Source: CAD feature listing. Evaluate the final solid. Frame: model axes, mm. Face numbers are marked on the shaded views. Coordinates: 2 decimals unless noted, no trailing zeros. Write item = value, one per line. Start each with the question number.
Autodesk Inventor part; units mm, degrees
ref_plane "YZ Plane" through (0, 0, 0) normal (1, 0, 0) x (0, 1, 0)
ref_plane "XZ Plane" through (0, 0, 0) normal (0, 1, 0) x (-1, 0, 0)
ref_plane "XY Plane" through (0, 0, 0) normal (0, 0, 1) x (1, 0, 0)
sketch "Esboço2" plane through (0, 0, 0) normal (0, 0, 1) x (1, 0, 0)
  line L0 (0, 0) -> (4, 0)
  line L1 (4, 0) -> (4, 4.3)
  line L2 (0, 4.3) -> (0, 0)
  arc A0 (0, 4.3) -> (4, 4.3) centre (2, 9.4235) ccw
  dimension "d0" = 4
  dimension "d1" = 4.3
  dimension "d70" = 5.5
revolve "Revolução1" add sketch "Esboço2" angle 360 about axis through (0, 0, 0) along (1, 0, 0)
sketch "Esboço11" plane through (4, 0, 0) normal (1, 0, 0) x (0, 0, -1)
  circle A0 centre (0, 0) radius 2.55
  circle A1 centre (0, 0) radius 2.95
  line L0 (0, 0) -> (2.95, 0)
  line L1 (2.55, 0) -> (2.5493, 0.06)
  line L2 (2.5493, 0.06) -> (2.55, 0)
  line L3 (2.55, 0) -> (2.5493, -0.06)
  line L4 (2.5493, 0.06) -> (2.9315, 0.3295)
  line L5 (2.5493, -0.06) -> (2.9315, -0.3295)
  line L6 (2.9315, 0.3295) -> (2.9255, 0.3791)
  line L7 (2.9315, -0.3295) -> (2.9255, -0.3791)
  line L8 (2.406, 0.8448) -> (2.6862, 1.2193)
  line L9 (2.4252, 0.788) -> (2.406, 0.8448)
  line L10 (2.4252, 0.788) -> (2.4431, 0.7307)
  line L11 (2.4431, 0.7307) -> (2.8899, 0.5925)
  circle A2 centre (0, 0) radius 2.95
  line L12 (2.6862, 1.2193) -> (2.6652, 1.2646)
  line L13 (2.8899, 0.5925) -> (2.8995, 0.5435)
  line L14 (2.0272, 1.547) -> (2.178, 1.9897)
  line L15 (2.063, 1.4989) -> (2.0272, 1.547)
  line L16 (2.063, 1.4989) -> (2.0977, 1.4499)
  line L17 (2.0977, 1.4499) -> (2.5653, 1.4566)
  circle A3 centre (0, 0) radius 2.95
  line L18 (2.178, 1.9897) -> (2.144, 2.0263)
  line L19 (2.5653, 1.4566) -> (2.5897, 1.4129)
  line L20 (1.4499, 2.0977) -> (1.4566, 2.5653)
  line L21 (1.4989, 2.063) -> (1.4499, 2.0977)
  line L22 (1.4989, 2.063) -> (1.547, 2.0272)
  line L23 (1.547, 2.0272) -> (1.9897, 2.178)
  circle A4 centre (0, 0) radius 2.95
  line L24 (1.4566, 2.5653) -> (1.4129, 2.5897)
  line L25 (1.9897, 2.178) -> (2.0263, 2.144)
  line L26 (0.7307, 2.4431) -> (0.5925, 2.8899)
  line L27 (0.788, 2.4252) -> (0.7307, 2.4431)
  line L28 (0.788, 2.4252) -> (0.8448, 2.406)
  line L29 (0.8448, 2.406) -> (1.2193, 2.6862)
  circle A5 centre (0, 0) radius 2.95
  line L30 (0.5925, 2.8899) -> (0.5435, 2.8995)
  line L31 (1.2193, 2.6862) -> (1.2646, 2.6652)
  line L32 (-0.06, 2.5493) -> (-0.3295, 2.9315)
  line L33 (0, 2.55) -> (-0.06, 2.5493)
  line L34 (0, 2.55) -> (0.06, 2.5493)
  line L35 (0.06, 2.5493) -> (0.3295, 2.9315)
  circle A6 centre (0, 0) radius 2.95
  line L36 (-0.3295, 2.9315) -> (-0.3791, 2.9255)
  line L37 (0.3295, 2.9315) -> (0.3791, 2.9255)
  line L38 (-0.8448, 2.406) -> (-1.2193, 2.6862)
  line L39 (-0.788, 2.4252) -> (-0.8448, 2.406)
  line L40 (-0.788, 2.4252) -> (-0.7307, 2.4431)
  line L41 (-0.7307, 2.4431) -> (-0.5925, 2.8899)
  circle A7 centre (0, 0) radius 2.95
  line L42 (-1.2193, 2.6862) -> (-1.2646, 2.6652)
  line L43 (-0.5925, 2.8899) -> (-0.5435, 2.8995)
  line L44 (-1.547, 2.0272) -> (-1.9897, 2.178)
  line L45 (-1.4989, 2.063) -> (-1.547, 2.0272)
  line L46 (-1.4989, 2.063) -> (-1.4499, 2.0977)
  line L47 (-1.4499, 2.0977) -> (-1.4566, 2.5653)
  circle A8 centre (0, 0) radius 2.95
  line L48 (-1.9897, 2.178) -> (-2.0263, 2.144)
  line L49 (-1.4566, 2.5653) -> (-1.4129, 2.5897)
  line L50 (-2.0977, 1.4499) -> (-2.5653, 1.4566)
  line L51 (-2.063, 1.4989) -> (-2.0977, 1.4499)
  line L52 (-2.063, 1.4989) -> (-2.0272, 1.547)
  line L53 (-2.0272, 1.547) -> (-2.178, 1.9897)
  circle A9 centre (0, 0) radius 2.95
  line L54 (-2.5653, 1.4566) -> (-2.5897, 1.4129)
  line L55 (-2.178, 1.9897) -> (-2.144, 2.0263)
  line L56 (-2.4431, 0.7307) -> (-2.8899, 0.5925)
  line L57 (-2.4252, 0.788) -> (-2.4431, 0.7307)
  line L58 (-2.4252, 0.788) -> (-2.406, 0.8448)
  line L59 (-2.406, 0.8448) -> (-2.6862, 1.2193)
  circle A10 centre (0, 0) radius 2.95
  line L60 (-2.8899, 0.5925) -> (-2.8995, 0.5435)
  line L61 (-2.6862, 1.2193) -> (-2.6652, 1.2646)
  line L62 (-2.5493, -0.06) -> (-2.9315, -0.3295)
  line L63 (-2.55, 0) -> (-2.5493, -0.06)
  line L64 (-2.55, 0) -> (-2.5493, 0.06)
  line L65 (-2.5493, 0.06) -> (-2.9315, 0.3295)
  circle A11 centre (0, 0) radius 2.95
  line L66 (-2.9315, -0.3295) -> (-2.9255, -0.3791)
  line L67 (-2.9315, 0.3295) -> (-2.9255, 0.3791)
  line L68 (-2.406, -0.8448) -> (-2.6862, -1.2193)
  line L69 (-2.4252, -0.788) -> (-2.406, -0.8448)
  line L70 (-2.4252, -0.788) -> (-2.4431, -0.7307)
  line L71 (-2.4431, -0.7307) -> (-2.8899, -0.5925)
  circle A12 centre (0, 0) radius 2.95
  line L72 (-2.6862, -1.2193) -> (-2.6652, -1.2646)
  line L73 (-2.8899, -0.5925) -> (-2.8995, -0.5435)
  line L74 (-2.0272, -1.547) -> (-2.178, -1.9897)
  line L75 (-2.063, -1.4989) -> (-2.0272, -1.547)
  line L76 (-2.063, -1.4989) -> (-2.0977, -1.4499)
  line L77 (-2.0977, -1.4499) -> (-2.5653, -1.4566)
  circle A13 centre (0, 0) radius 2.95
  line L78 (-2.178, -1.9897) -> (-2.144, -2.0263)
  line L79 (-2.5653, -1.4566) -> (-2.5897, -1.4129)
  line L80 (-1.4499, -2.0977) -> (-1.4566, -2.5653)
  line L81 (-1.4989, -2.063) -> (-1.4499, -2.0977)
  line L82 (-1.4989, -2.063) -> (-1.547, -2.0272)
  line L83 (-1.547, -2.0272) -> (-1.9897, -2.178)
  circle A14 centre (0, 0) radius 2.95
  line L84 (-1.4566, -2.5653) -> (-1.4129, -2.5897)
  line L85 (-1.9897, -2.178) -> (-2.0263, -2.144)
  line L86 (-0.7307, -2.4431) -> (-0.5925, -2.8899)
  line L87 (-0.788, -2.4252) -> (-0.7307, -2.4431)
  line L88 (-0.788, -2.4252) -> (-0.8448, -2.406)
  line L89 (-0.8448, -2.406) -> (-1.2193, -2.6862)
  circle A15 centre (0, 0) radius 2.95
  line L90 (-0.5925, -2.8899) -> (-0.5435, -2.8995)
  line L91 (-1.2193, -2.6862) -> (-1.2646, -2.6652)
  line L92 (0.06, -2.5493) -> (0.3295, -2.9315)
  line L93 (0, -2.55) -> (0.06, -2.5493)
  line L94 (0, -2.55) -> (-0.06, -2.5493)
  line L95 (-0.06, -2.5493) -> (-0.3295, -2.9315)
  circle A16 centre (0, 0) radius 2.95
  line L96 (0.3295, -2.9315) -> (0.3791, -2.9255)
  line L97 (-0.3295, -2.9315) -> (-0.3791, -2.9255)
  line L98 (0.8448, -2.406) -> (1.2193, -2.6862)
  line L99 (0.788, -2.4252) -> (0.8448, -2.406)
  line L100 (0.788, -2.4252) -> (0.7307, -2.4431)
  line L101 (0.7307, -2.4431) -> (0.5925, -2.8899)
  circle A17 centre (0, 0) radius 2.95
  line L102 (1.2193, -2.6862) -> (1.2646, -2.6652)
  line L103 (0.5925, -2.8899) -> (0.5435, -2.8995)
  line L104 (1.547, -2.0272) -> (1.9897, -2.178)
  line L105 (1.4989, -2.063) -> (1.547, -2.0272)
  line L106 (1.4989, -2.063) -> (1.4499, -2.0977)
  line L107 (1.4499, -2.0977) -> (1.4566, -2.5653)
  circle A18 centre (0, 0) radius 2.95
  line L108 (1.9897, -2.178) -> (2.0263, -2.144)
  line L109 (1.4566, -2.5653) -> (1.4129, -2.5897)
  line L110 (2.0977, -1.4499) -> (2.5653, -1.4566)
  line L111 (2.063, -1.4989) -> (2.0977, -1.4499)
  line L112 (2.063, -1.4989) -> (2.0272, -1.547)
  line L113 (2.0272, -1.547) -> (2.178, -1.9897)
  circle A19 centre (0, 0) radius 2.95
  line L114 (2.5653, -1.4566) -> (2.5897, -1.4129)
  line L115 (2.178, -1.9897) -> (2.144, -2.0263)
  line L116 (2.4431, -0.7307) -> (2.8899, -0.5925)
  line L117 (2.4252, -0.788) -> (2.4431, -0.7307)
  line L118 (2.4252, -0.788) -> (2.406, -0.8448)
  line L119 (2.406, -0.8448) -> (2.6862, -1.2193)
  circle A20 centre (0, 0) radius 2.95
  line L120 (2.8899, -0.5925) -> (2.8995, -0.5435)
  line L121 (2.6862, -1.2193) -> (2.6652, -1.2646)
  point P0 (2.8056, 0.9116)
  point P1 (2.3866, 1.734)
  point P2 (1.734, 2.3866)
  point P3 (0.9116, 2.8056)
  point P4 (0, 2.95)
  point P5 (-0.9116, 2.8056)
  point P6 (-1.734, 2.3866)
  point P7 (-2.3866, 1.734)
  point P8 (-2.8056, 0.9116)
  point P9 (-2.95, 0)
  point P10 (-2.8056, -0.9116)
  point P11 (-2.3866, -1.734)
  point P12 (-1.734, -2.3866)
  point P13 (-0.9116, -2.8056)
  point P14 (0, -2.95)
  point P15 (0.9116, -2.8056)
  point P16 (1.734, -2.3866)
  point P17 (2.3866, -1.734)
  point P18 (2.8056, -0.9116)
  dimension "d59" = 5.9
  dimension "d58" = 5.1
  dimension "d60" = 0.06
  dimension "d61" = 0.06
  dimension "d62" = 0.05
  dimension "d63" = 0.05
  dimension "d66" = 360
extrude "Extrusão5" cut sketch "Esboço11" against normal blind 3.5 contours A0 | A0 L11 A1 L4 | L5 A1 L116 A0 | A0 L17 A1 L8 | L119 A1 L110 A0 | A0 L23 A1 L14 | L113 A1 L104 A0 | A0 L29 A1 L20 | L107 A1 L98 A0 | A0 L35 A1 L26 | L101 A1 L92 A0 | A0 L41 A1 L32 | L95 A1 L86 A0 | A0 L47 A1 L38 | L89 A1 L80 A0 | A0 L53 A1 L44 | L83 A1 L74 A0 | A0 L59 A1 L50 | L77 A1 L68 A0 | A0 L65 A1 L56 | L71 A1 L62 A0
sketch "Esboço12" plane through (4, 0, 0) normal (1, 0, 0) x (0, 0, -1)
  point P0 (0, 0)
sketch "Esboço13" plane through (0.5, 0, 0) normal (1, 0, 0) x (0, 0, -1)
  point P0 (0, 0)
properties part number "roda corda"
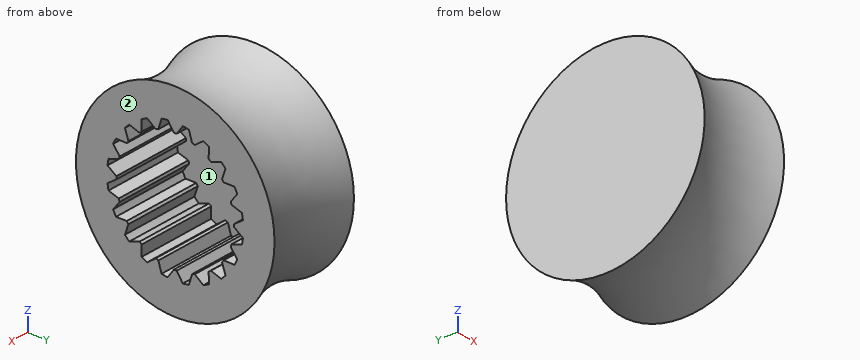
Item 1: First-contact query: pin 1 (2 mm diameter, centred on x = 2.5, z = 1.5, fed in from -Y); pin 2 (1 mm diameter, centred on x = 2.5, z = 2.5, fed in from +Y); pin 3 (1 mm diameter, centred on x = 2.5, y = 1.5, fed in from +Z). Flat tips, straight axial feed; report the tip coordinate or a pass-through.
Item 2: Draft query along Y for the marked faces 1 and 2. Return one class per face: released by +Y, released by -Y, zero draft, split by the parting line, or undercut.
Item 3: Material intervals for L1, parallel to Z at x = 3.05, y = 2.5; L2, parallel to Z at x = 2.9, y = 2.5; L3, parallel to X at y = 1, z = 1, sorted ascending. Write a range as [from, to].
Responses:
q1.pin_1 = -3.98
q1.pin_2 = 3.41
q1.pin_3 = 3.83
q2.face_1 = undercut
q2.face_2 = zero draft
q3.L1 = [-3.15, -1.46], [-0.97, -0.71], [0.71, 0.97], [1.46, 3.15]
q3.L2 = [-3.12, -1.46], [-0.97, -0.71], [0.71, 0.97], [1.46, 3.12]
q3.L3 = [0, 0.5]
